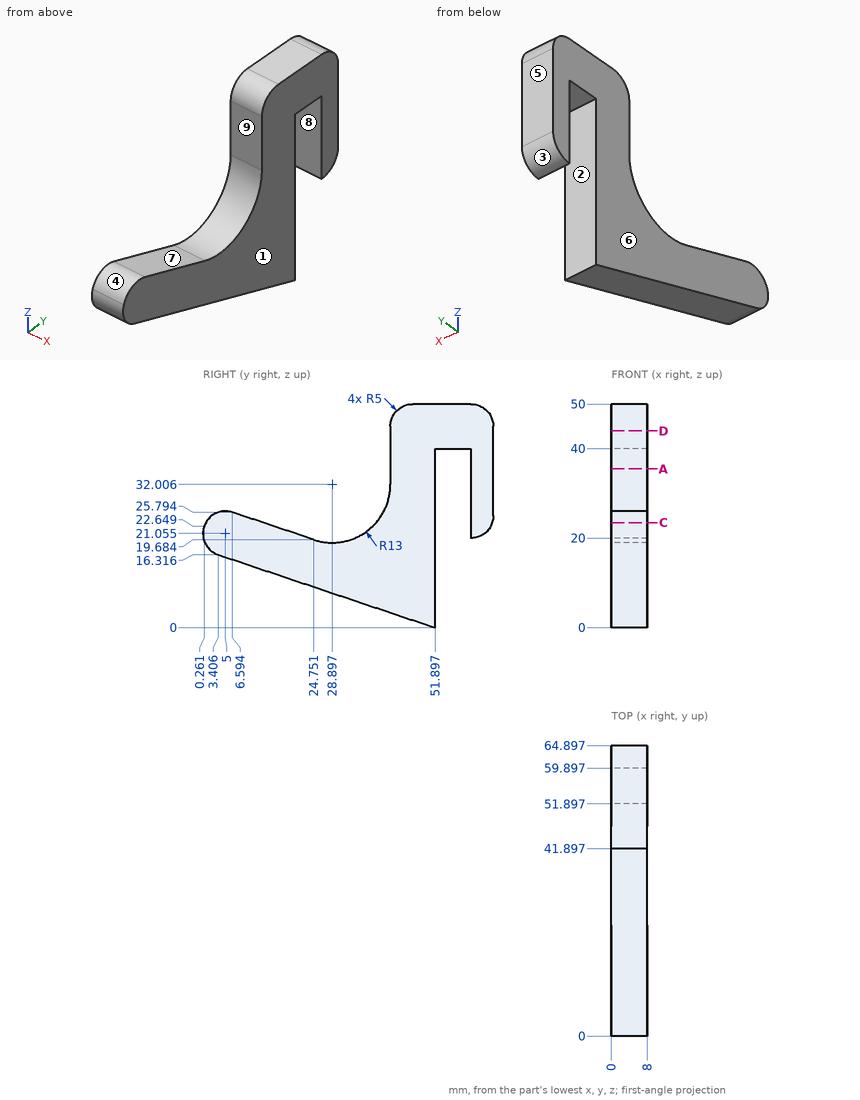
Here's the drawing with two shaded views (mm, measured from the low corner). I have some questions. A direction names the side the tool comes from. Give positions to 0.01 mm unless a question says otherwise; leave off trailing zeros. Write each loop counter-clockwise with the first axis right and the second up, starting at its lowest first coordinate (ties: lowest second). Pieces come first, ordered by that corner, then holes. Notation, with made-up numbers: (85.5, 58) -> (131.5, 58) arc R3 cw to (131.5, 63) -> close; hole circle Ø2 at (-2.75, 50.5). An arc over 180 degrees is marked (long way). Use one line per item in the form item = value. Start each with the question number.
1. Thinking about a two-plate mould opening in Y: for the marked faces 1, 2, 3 and 4, which applies, +Y half, -Y half, draft (parallel to the pull), parting line (faces both ways), or undercut?
2. Will these pins go through, and if not, where does the flat tip stop? pin 1 Ø3 at (x, y) = (6.5, 21) entering from +Z; pin 2 Ø4 at (y, z) = (43, 38.5) entering from -X; pin 3 Ø4 at (x, y) = (5, 55) entering from -Z; pin 4 Ø4 at (x, z) = (4, 18) entering from -Y.
3. On a 3-axis mill with a long thin cutter (end or side, diameter ignored), from which of +Z, -Z, +X, -X, +Y, -Y can I reach the whole of each face in a straight line? I mean the marked faces 5, 6, 7, 8 and 9. Say none if no direction works.
4. Imagine slicing it at C-C on z = 23.5. List the corners of the cut face in (x, y) for me, plus the area to 3 significant figures.
5. Imagine slicing it at A-A on z = 35.5. List the corners of the cut face in (x, y) for me, plus the area to 3 significant figures.
6. If I drill on L1, parallel to Y at x = 2, z = 33; L2, parallel to Z at x = 6.5, y = 58.5; L3, parallel to Y at x = 5.75, z = 45, over which ranges is the centre line in solid material (lowest first)?
7. Imagine slicing it at D-D on z = 44. List the corners of the cut face in (x, y) for me, plus the area to 3 significant figures.
Entries:
q1.face_1 = draft
q1.face_2 = undercut
q1.face_3 = +Y half
q1.face_4 = undercut
q2.pin_1 = 21.45
q2.pin_2 = 0
q2.pin_3 = 40
q2.pin_4 = 0.11
q3.face_5 = +Z, -Z, +X, -X, +Y
q3.face_6 = +Z, -Z, -X, +Y, -Y
q3.face_7 = +Z, +X, -X
q3.face_8 = -Z, +X, -X
q3.face_9 = +Z, +X, -X, -Y
q4.outline = (0, 0.64) -> (8, 0.64) -> (8, 13.41) -> (0, 13.41) -> close; (0, 38.73) -> (8, 38.73) -> (8, 51.9) -> (0, 51.9) -> close; (0, 59.9) -> (8, 59.9) -> (8, 64.67) -> (0, 64.67) -> close
q4.area = 246 mm²
q5.outline = (0, 41.9) -> (8, 41.9) -> (8, 51.9) -> (0, 51.9) -> close; (0, 59.9) -> (8, 59.9) -> (8, 64.9) -> (0, 64.9) -> close
q5.area = 120 mm²
q6.L1 = 41.9 to 51.9, 59.9 to 64.9
q6.L2 = 40 to 50
q6.L3 = 41.9 to 64.9
q7.outline = (0, 41.9) -> (8, 41.9) -> (8, 64.9) -> (0, 64.9) -> close
q7.area = 184 mm²
